from build123d import *

# Parameters (mm, degrees)
EXTRUDE_1_DEPTH     = 30
SHELL_START         = 5
SHELL_1_DEPTH       = 25
SKETCH_3_W          = 31.232058984
SKETCH_3_H          = 30.58107444
CUT_EXTRUDE_1_DEPTH = 25


# Read off the part's stored shape, not the designer's step: 抽壳1
with BuildPart() as part:
    # 草图1 → 凸台-拉伸1 (new body)
    with BuildSketch(Plane(origin=(0, 0, 0), x_dir=(1, 0, 0), z_dir=(0, 1, 0))):
        with BuildLine():
            Line((-40, -27), (-40, -25))
            Line((-40, -25), (-38, -25))
            Line((-38, -25), (-38, -19))
            Line((-38, -19), (-30, -19))
            Line((-30, -19), (-30, 19))
            Line((-30, 19), (-38, 19))
            Line((-38, 19), (-38, 25))
            Line((-38, 25), (-40, 25))
            Line((-40, 25), (-40, 27))
            ThreePointArc((-40, 27), (0, 48.259714048), (40, 27))
            Line((40, 27), (40, 25))
            Line((40, 25), (38, 25))
            Line((38, 25), (38, 19))
            Line((38, 19), (30, 19))
            Line((30, 19), (30, -19))
            Line((30, -19), (38, -19))
            Line((38, -19), (38, -25))
            Line((38, -25), (40, -25))
            Line((40, -25), (40, -27))
            ThreePointArc((40, -27), (0, -48.259714048), (-40, -27))
        make_face()
    extrude(amount=EXTRUDE_1_DEPTH)

    # 抽壳1 outline → 抽壳1 (cut)
    with BuildSketch(Plane(origin=(0, 0, 0), x_dir=(1, 0, 0), z_dir=(0, 1, 0)).offset(SHELL_START)):
        with BuildLine():
            Line((-33, -24), (-33, -27.971465094))
            ThreePointArc((-33, -27.971465094), (0, -43.259714048), (33, -27.971465094))
            Line((33, -27.971465094), (33, -24))
            Line((33, -24), (25, -24))
            Line((25, -24), (25, 24))
            Line((25, 24), (33, 24))
            Line((33, 24), (33, 27.971465094))
            ThreePointArc((33, 27.971465094), (0, 43.259714048), (-33, 27.971465094))
            Line((-33, 27.971465094), (-33, 24))
            Line((-33, 24), (-25, 24))
            Line((-25, 24), (-25, -24))
            Line((-25, -24), (-33, -24))
        make_face()
    extrude(amount=SHELL_1_DEPTH, mode=Mode.SUBTRACT)

    # 草图3 → 切除-拉伸1 (cut)
    with BuildSketch(Plane.XZ):
        with BuildLine():
            Line((-30, 29.393876913), (-30, 37.802116343))
            ThreePointArc((-30, 37.802116343), (0, 48.259714048), (30, 37.802116343))
            Line((30, 37.802116343), (30, 29.393876913))
            ThreePointArc((30, 29.393876913), (0, 42), (-30, 29.393876913))
        make_face()
        with BuildLine():
            Line((-30, -29.393876913), (-30, -37.802116343))
            ThreePointArc((-30, -37.802116343), (0, -48.259714048), (30, -37.802116343))
            Line((30, -37.802116343), (30, -29.393876913))
            ThreePointArc((30, -29.393876913), (0, -42), (-30, -29.393876913))
        make_face()
        Rectangle(SKETCH_3_W, SKETCH_3_H)
    extrude(amount=-CUT_EXTRUDE_1_DEPTH, mode=Mode.SUBTRACT)


solid = part.part
Can you work these out from the model? Positions are in its coordinate system, mm. A direction names the side the tool comes from. Round coordinates to 2 decimals unless told otherwise and drop trailing zeros. Write each loop counter-clockwise with the first axis right and the second up, starting at its lowest first coordinate (ties: lowest second). Pieces come first, ordered by that corner, then holes. Notation, with made-up numbers: (45, 20.25) - (64, 20.25) arc R16 ccw to (64, 45.25) - close; hole circle Ø10 at (-23, 53.25). An arc over 180 degrees is marked (long way). Write each question's results on one line, items separated by ' | '. Start each with the question number.
1) Please list where these lines run through material, in increasing order: line 1 (X direction, y = 15.25, z = 2.5); line 2 (X direction, y = 14.75, z = 23); line 3 (Z direction, x = -31, y = 19.5).
2) Suppose I cut it at B-B (z = -3). List the corners of the cut face in (x, y) for me, and give its area (3 significant figures).
3) Suppose I cut it at C-C (x = -4). List the corners of the cut face in (y, z) for me.
4) Which directions (+Z, -Z, +X, -X, +Y, -Y) give clear straight access to the entire face, cutting with the end or side of a thin tool? Please do faces 1 (the flat face through (0, 2, -15.291)), 2 (the cylindrical face through (-0.18, 26.7, 43.26)), 3 (the flat face through (-39, 15, 25)), 4 (the flat face through (38, 15, 22)).
5) We'd pull the mould along Z, two halves only. Please class faces 5 (the flat face through (0, 25, 44)), 6 (the flat face through (-15.616, 2, 0)), 7 (the flat face through (30, 15, 0)): released by +Z, released by -Z, zero draft, split by the parting line, or undercut.
6) Suppose I cut it at D-D (x = -21). List the corners of the cut face in (y, z) for me.
7) For pin 1 Ø4 at (y, z) = (14.5, -32) entering from +X; pin 2 Ø12 at (x, y) = (21.5, 5) entering from -Z; pin 3 Ø10 at (x, z) = (1.5, 30) entering from +Y, each with a flat end and sliding along its axis, tell me the tip position at first contact or that it passes through.
Here are the results:
1) line 1: x = -30 to -25, 25 to 30 | line 2: x = -38 to -25, 25 to 38 | line 3: z = -36.99 to -30.17, -24 to -19, 19 to 24, 30.17 to 36.99
2) outline: (-30, 0) - (-15.62, 0) - (-15.62, 5) - (-25, 5) - (-25, 30) - (-30, 30) - close; (15.62, 0) - (30, 0) - (30, 30) - (25, 30) - (25, 5) - (15.62, 5) - close | area: 394 mm2
3) outline: (0, -41.81) - (5, -41.81) - (5, -15.29) - (0, -15.29) - close; (0, 15.29) - (5, 15.29) - (5, 41.81) - (0, 41.81) - close; (25, -48.09) - (30, -48.09) - (30, -43.07) - (25, -43.07) - close; (25, 43.07) - (30, 43.07) - (30, 48.09) - (25, 48.09) - close
4) face 1: +Y, -Y | face 2: +Y | face 3: -X, +Y, -Y | face 4: +X, +Y, -Y
5) face 5: zero draft | face 6: undercut | face 7: undercut
6) outline: (0, -36.37) - (5, -36.37) - (5, 36.37) - (0, 36.37) - close; (25, -43.45) - (30, -43.45) - (30, -37.82) - (25, -37.82) - close; (25, 37.82) - (30, 37.82) - (30, 43.45) - (25, 43.45) - close
7) pin 1: stops at x = 37.8 | pin 2: stops at z = -39.04 | pin 3: stops at y = 5
